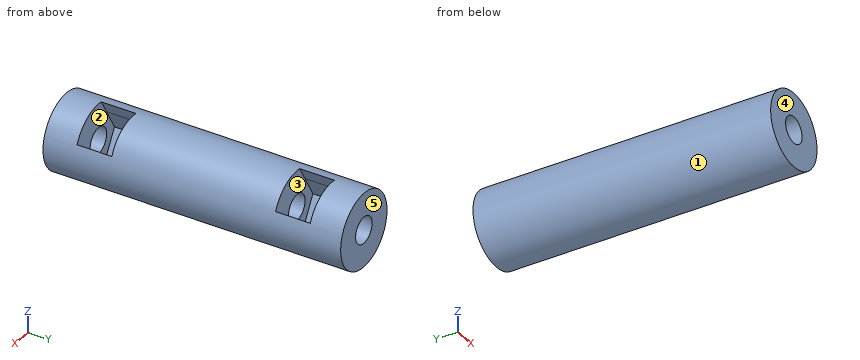
```python
from build123d import *

# Parameters (mm, degrees)
SKETCH1_R           = 9.525
BOSS_EXTRUDE1_DEPTH = 38.1
CUT_EXTRUDE1_DEPTH  = 4.445
SKETCH3_R           = 3.3782
CUT_EXTRUDE2_DEPTH  = 78.381465804


with BuildPart() as part:
    # Sketch1 → Boss-Extrude1 (new, symmetric)
    with BuildSketch(Plane(origin=(0, 0, 0), x_dir=(1, 0, 0), z_dir=(0, 1, 0))):
        with Locations(Location((0, 0, 0), (0, 0, 90))):
            Circle(SKETCH1_R)
    extrude(amount=BOSS_EXTRUDE1_DEPTH, both=True)

    # Sketch2 → Cut-Extrude1 (cut, symmetric)
    with BuildSketch(Plane(origin=(0, -25.4, 0), x_dir=(-1, 0, 0), z_dir=(0, -1, 0))):
        Polygon((-3.299556788, 5.715), (-6.599113577, 0), (6.599113577, 0), (3.299556788, 5.715), align=None)
        Polygon((6.599113577, 0), (-6.599113577, 0), (-3.299556788, -5.715), (3.299556788, -5.715), align=None)
        with BuildLine():
            ThreePointArc((1.139335183, -9.456613577), (-4.7625, -8.248891971), (-8.759335183, -3.741613577))
            Line((-8.759335183, -3.741613577), (-6.599113577, 0))
            Line((-6.599113577, 0), (-3.299556788, -5.715))
            Line((-3.299556788, -5.715), (3.299556788, -5.715))
            Line((3.299556788, -5.715), (1.139335183, -9.456613577))
        make_face()
    cut_extrude1 = extrude(amount=CUT_EXTRUDE1_DEPTH, both=True, mode=Mode.SUBTRACT)

    # Mirror1: Cut-Extrude1 across plane
    add(cut_extrude1.mirror(Plane.ZX), mode=Mode.SUBTRACT)

    # Sketch3 → Cut-Extrude2 (cut, through all)
    with BuildSketch(Plane(origin=(0, 38.1, 0), x_dir=(1, 0, 0), z_dir=(0, 1, 0))):
        with Locations(Location((0, 0, 0), (0, 0, 270))):
            Circle(SKETCH3_R)
    extrude(amount=-CUT_EXTRUDE2_DEPTH, mode=Mode.SUBTRACT)


solid = part.part
```
Source: CAD feature listing. Evaluate the final solid. Frame: model axes, mm. Face numbers are marked on the shaded views. A direction names the side the tool comes from. Give positions to 0.01 mm unless a question says otherwise; leave off trailing zeros. Order: outer loops, then holes, each group sorted by start corner. A loop starts at its lowest first (then second) coordinate and runs counter-clockwise, first axis right, second up.
(1) Material intervals for line 1 along Y through (x, z) = (-4, -2) (3 decimals); line 2 along X through (y, z) = (7, 0) (3 decimals); line 3 along Z through (x, y) = (0.5, -8.5), sorted ascending.
(2) Pull-direction query (Y, two-part tool) for the marked faces 3, 4 and 5; classes: +Y half, -Y half, draft (parallel to the pull), parting line (faces both ways), or undercut.
(3) Section query B-B (z = -1.5). Return the cut outline in (x, y) (3 decimals).
(4) Section query A-A (x = 0). Return the cut outline in (y, z) (3 decimals).
(5) Section query C-C (y = -11). Return the cut outline in (x, z) (3 decimals).
(6) Section query D-D (z = 8). Return the cut outline in (x, y) (3 decimals).
(7) Access query for the marked faces 1 and 2. Directions: +Z, -Z, +X, -X, +Y, -Y. A direction counts if a zero-diameter tool reaches every point of the face in a straight line with its end or side. Return the directions, or none.
(8) Contact query for flat-ended pins moving along their axis: P1, Ø1, axis at y = -9, z = 2.5, coming from the -X side; P2, Ø8, axis at x = 5.5, y = 7.5, coming from the -Z side; P3, Ø1, axis at y = 8.5, z = 1, coming from the +X side; P4, Ø5.5, axis at x = 0, z = 0, coming from the +Y side. Output: stop coordinate, or through.
Outcome:
1. line 1: y = -38.1 to -29.845, -20.955 to 20.955, 29.845 to 38.1
1. line 2: x = -9.525 to -3.378, 3.378 to 9.525
1. line 3: z = -9.51 to -3.34, 3.34 to 9.51
2. face 3: undercut
2. face 4: -Y half
2. face 5: +Y half
3. outline: (-9.406, -38.1) - (-3.027, -38.1) - (-3.027, -29.845) - (-5.733, -29.845) - (-5.733, -20.955) - (-3.027, -20.955) - (-3.027, 20.955) - (-5.733, 20.955) - (-5.733, 29.845) - (-3.027, 29.845) - (-3.027, 38.1) - (-9.406, 38.1) - close; (3.027, -38.1) - (9.406, -38.1) - (9.406, 38.1) - (3.027, 38.1) - (3.027, 29.845) - (5.733, 29.845) - (5.733, 20.955) - (3.027, 20.955) - (3.027, -20.955) - (5.733, -20.955) - (5.733, -29.845) - (3.027, -29.845) - close
4. outline: (-38.1, -9.525) - (38.1, -9.525) - (38.1, -3.378) - (29.845, -3.378) - (29.845, -5.715) - (20.955, -5.715) - (20.955, -3.378) - (-20.955, -3.378) - (-20.955, -5.715) - (-29.845, -5.715) - (-29.845, -3.378) - (-38.1, -3.378) - close; (-38.1, 3.378) - (-29.845, 3.378) - (-29.845, 9.525) - (-38.1, 9.525) - close; (-20.955, 3.378) - (20.955, 3.378) - (20.955, 9.525) - (-20.955, 9.525) - close; (29.845, 3.378) - (38.1, 3.378) - (38.1, 9.525) - (29.845, 9.525) - close
5. outline: circle Ø19.05 at (0, 0); hole circle Ø6.756 at (0, 0)
6. outline: (-5.17, -38.1) - (5.17, -38.1) - (5.17, -29.845) - (-1.98, -29.845) - (-1.98, -20.955) - (5.17, -20.955) - (5.17, 20.955) - (-1.98, 20.955) - (-1.98, 29.845) - (5.17, 29.845) - (5.17, 38.1) - (-5.17, 38.1) - close
7. face 1: +Y, -Y
7. face 2: none
8. P1: stops at x = -9.31
8. P2: stops at z = -9.41
8. P3: stops at x = 9.51
8. P4: passes through
